```python
from build123d import *

# Parameters (mm, degrees)
SKETCH1_R           = 6.35
SKETCH1_R_2         = 4.7625
BOSS_EXTRUDE1_DEPTH = 3.175
SKETCH1_3_R         = 4.7625
SKETCH1_3_R_2       = 3.475
BOSS_EXTRUDE2_DEPTH = 10.9
CHAMFER1_SIZE       = 3


with BuildPart() as part:
    # Sketch1 → Boss-Extrude1 (new body)
    with BuildSketch(Plane(origin=(0, 0, 0), x_dir=(1, 0, 0), z_dir=(0, 1, 0))):
        with Locations(Location((0, 0, 0), (0, 0, 270))):
            Circle(SKETCH1_R)
        with Locations(Location((0, 0, 0), (0, 0, 270))):
            Circle(SKETCH1_R_2, mode=Mode.SUBTRACT)
    extrude(amount=BOSS_EXTRUDE1_DEPTH)

    # Sketch1<3> → Boss-Extrude2 (add)
    with BuildSketch(Plane(origin=(0, 0, 0), x_dir=(1, 0, 0), z_dir=(0, 1, 0))):
        with Locations(Location((0, 0, 0), (0, 0, 270))):
            Circle(SKETCH1_3_R)
        with Locations(Location((0, 0, 0), (0, 0, 270))):
            Circle(SKETCH1_3_R_2, mode=Mode.SUBTRACT)
    extrude(amount=BOSS_EXTRUDE2_DEPTH)

    # Chamfer1
    # the kernel refuses this chamfer: 3 mm, written as the material it adds along each edge
    with BuildSketch(Plane(origin=(0, 3.175, 0), x_dir=(0, 0, 1), z_dir=(-1, 0, 0))) as chamfer1_piece_1_section:
        Polygon((4.7625 + CHAMFER1_SIZE, 0), (4.7625, CHAMFER1_SIZE), (4.7625, 0), align=None)
    chamfer1_piece_1 = revolve(axis=Axis((0, 3.175, 0), (0, 1, 0)), mode=Mode.PRIVATE)
    chamfer1_piece_1 = chamfer1_piece_1 & Plane(origin=(0, 5.38786909, 0), x_dir=(0, 0, 1), z_dir=(0, -1, 0)) * Cylinder(6.35, 32, mode=Mode.PRIVATE)
    add(chamfer1_piece_1)


solid = part.part
```
The listing builds one solid part. Answer for the finished solid, in the listing's coordinates (mm). Round coordinates to 2 decimals unless told otherwise and drop trailing zeros. Order: outer loops, then holes, each group sorted by start corner. A loop starts at its lowest first (then second) coordinate and runs counter-clockwise, first axis right, second up. Notation, with made-up numbers: (50.25, 62) - (90.25, 62) arc R10 ccw to (90.25, 72) - close; hole circle Ø4 at (77, 64.5). An arc over 180 degrees is marked (long way). Put each result on its own line as item: value. Start each with the question number.
(1) Given P1, Ø3, axis at x = -4, y = 2, coming from the -Z side; P2, Ø5.5, axis at x = 0, z = 0, coming from the +Y side; P3, Ø5, axis at y = 9.5, z = 1, coming from the +X side; P4, Ø1.5, axis at x = -5, z = -3, coming from the +Y side, each flat-ended and moving along its own axis, determine where each tip first touches the part or whether it passes through.
(2) Find section C-C (y = 0.5). Give the vertices of the cut face in (x, z) (3 decimals).
(3) Determine the mould class of faces 1 (the flat face through (-3, 0, 3)), 2 (the cylindrical face through (-2.9, 8.5, -3.78)), 3 (the cylindrical face through (-3.392, 5.374, -0.753)) for opening direction Z: released by +Z, released by -Z, zero draft, split by the parting line, or undercut.
(4) Straight lines are drawn through the part: probe 1 along X at (y, z) = (7.5, 0) (1 decimal); probe 2 along X at (y, z) = (4.5, 0) (3 decimals); probe 3 along Z at (x, y) = (1, 4). For each, find the intervals that lie inside material, in ascending order. Write a range as from..to.
Reply:
1. P1: z = -5.84
1. P2: through
1. P3: x = 4.76
1. P4: y = 5.86
2. outline: circle Ø12.7 at (0, 0); hole circle Ø6.95 at (0, 0)
3. face 1: zero draft
3. face 2: split by the parting line
3. face 3: undercut
4. probe 1: -4.8..-3.5, 3.5..4.8
4. probe 2: -6.35..-3.475, 3.475..6.35
4. probe 3: -6.27..-3.33, 3.33..6.27
